Here's how the part is built. I have some questions about the finished solid (model axes, mm). Face numbers are marked on the shaded views. Coordinates: 2 decimals unless noted, no trailing zeros. Write each loop counter-clockwise with the first axis right and the second up, starting at its lowest first coordinate (ties: lowest second). Pieces come first, ordered by that corner, then holes.
Item 1: Please list where these lines run through material, in increasing order: line 1 (X direction, y = 1, z = 51); line 2 (X direction, y = 17.5, z = 131); line 3 (Y direction, x = -18, z = 156).
Item 2: If we mould it in two halves opening along X, with no side actions, what happens to the marked faces 1 and 2? For each: pulls with the +X half, pulls with the -X half, needs draft (parallel to the pull), parting line crosses it, or undercut.
Item 3: I'm going to push flat-ended pins straight in: P1, Ø1.2, axis at y = -18, z = 160, coming from the +X side; P2, Ø12, axis at x = 2.5, y = -11.5, coming from the +Z side; P3, Ø1, axis at x = 11, z = 162.5, coming from the +Y side. Where does each tip first touch, or does it pass through?
Item 4: I want a section at C-C (y = 19). Please give me the cut outline in (x, z), and give its area (3 significant figures).
Item 5: I want a section at B-B (x = 0). Please give me the cut outline in (y, z), and give its area (3 significant figures).
Item 6: I want a section at A-A (y = 1.5). Please give me the cut outline in (x, z), and give its area (3 significant figures).
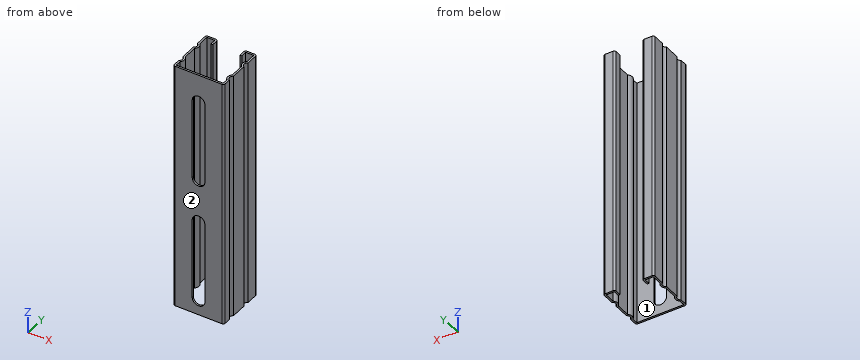
from build123d import *

# Parameters (mm, degrees)
BASE_EXTRUDE_DEPTH = 203.2
SLOT_DEPTH         = 227.830922417
LPATTERN1_COUNT    = 2
LPATTERN1_PITCH    = 101.6


with BuildPart() as part:
    # Sketch1 → Base-Extrude (new body)
    with BuildSketch(Plane.XY):
        with BuildLine():
            Line((-20.6375, 21.1074), (-20.6375, 11.73965134))
            ThreePointArc((-20.6375, 11.73965134), (-19.1389, 9.144), (-20.6375, 6.54834866))
            Line((-20.6375, 6.54834866), (-20.6375, -6.54834866))
            ThreePointArc((-20.6375, -6.54834866), (-19.1389, -9.144), (-20.6375, -11.73965134))
            Line((-20.6375, -11.73965134), (-20.6375, -17.1704))
            ThreePointArc((-20.6375, -17.1704), (-20.198570222, -18.230070222), (-19.1389, -18.669))
            Line((-19.1389, -18.669), (19.1389, -18.669))
            ThreePointArc((19.1389, -18.669), (20.198570222, -18.230070222), (20.6375, -17.1704))
            Line((20.6375, -17.1704), (20.6375, -11.73965134))
            ThreePointArc((20.6375, -11.73965134), (19.1389, -9.144), (20.6375, -6.54834866))
            Line((20.6375, -6.54834866), (20.6375, 6.54834866))
            ThreePointArc((20.6375, 6.54834866), (19.1389, 9.144), (20.6375, 11.73965134))
            Line((20.6375, 11.73965134), (20.6375, 21.1074))
            ThreePointArc((20.6375, 21.1074), (20.198570222, 22.167070222), (19.1389, 22.606))
            Line((19.1389, 22.606), (12.6111, 22.606))
            ThreePointArc((12.6111, 22.606), (11.551429778, 22.167070222), (11.1125, 21.1074))
            Line((11.1125, 21.1074), (11.1125, 16.256))
            Line((11.1125, 16.256), (12.6111, 16.256))
            Line((12.6111, 16.256), (12.6111, 21.1074))
            Line((12.6111, 21.1074), (19.1389, 21.1074))
            Line((19.1389, 21.1074), (19.1389, 12.494971471))
            ThreePointArc((19.1389, 12.494971471), (17.6403, 9.144), (19.1389, 5.793028529))
            Line((19.1389, 5.793028529), (19.1389, -5.793028529))
            ThreePointArc((19.1389, -5.793028529), (17.6403, -9.144), (19.1389, -12.494971471))
            Line((19.1389, -12.494971471), (19.1389, -17.1704))
            Line((19.1389, -17.1704), (-19.1389, -17.1704))
            Line((-19.1389, -17.1704), (-19.1389, -12.494971471))
            ThreePointArc((-19.1389, -12.494971471), (-17.6403, -9.144), (-19.1389, -5.793028529))
            Line((-19.1389, -5.793028529), (-19.1389, 5.793028529))
            ThreePointArc((-19.1389, 5.793028529), (-17.6403, 9.144), (-19.1389, 12.494971471))
            Line((-19.1389, 12.494971471), (-19.1389, 21.1074))
            Line((-19.1389, 21.1074), (-12.6111, 21.1074))
            Line((-12.6111, 21.1074), (-12.6111, 16.256))
            Line((-12.6111, 16.256), (-11.1125, 16.256))
            Line((-11.1125, 16.256), (-11.1125, 21.1074))
            ThreePointArc((-11.1125, 21.1074), (-11.551429778, 22.167070222), (-12.6111, 22.606))
            Line((-12.6111, 22.606), (-19.1389, 22.606))
            ThreePointArc((-19.1389, 22.606), (-20.198570222, 22.167070222), (-20.6375, 21.1074))
        make_face()
    extrude(amount=BASE_EXTRUDE_DEPTH)

    # Sketch2 → Slot (cut, through all)
    with BuildSketch(Plane(origin=(1.121412804, -18.669, -18.780160044), x_dir=(1, 0, 0), z_dir=(0, -1, 0))):
        with BuildLine():
            Line((4.037962196, 97.361410044), (4.037962196, 31.480160044))
            ThreePointArc((4.037962196, 31.480160044), (-1.121412804, 26.320785044), (-6.280787804, 31.480160044))
            Line((-6.280787804, 31.480160044), (-6.280787804, 97.361410044))
            ThreePointArc((-6.280787804, 97.361410044), (-1.121412804, 102.520785044), (4.037962196, 97.361410044))
        make_face()
    slot = extrude(amount=-SLOT_DEPTH, mode=Mode.SUBTRACT)

    # LPattern1: Slot ×2
    with Locations(*[(0, 0, i * LPATTERN1_PITCH) for i in range(1, LPATTERN1_COUNT)]):
        add(slot, mode=Mode.SUBTRACT)


solid = part.part
Answer:
1. line 1: x = -20.64 to -19.14, 19.14 to 20.64
1. line 2: x = -20.64 to -19.14, -12.61 to -11.11, 11.11 to 12.61, 19.14 to 20.64
1. line 3: y = -18.67 to -17.17, -10.91 to -7.38, 7.38 to 10.91, 21.11 to 22.61
2. face 1: undercut
2. face 2: needs draft
3. P1: stops at x = 20.62
3. P2: stops at z = 203.2
3. P3: stops at y = 22.11
4. outline: (-20.64, 0) - (-19.14, 0) - (-19.14, 203.2) - (-20.64, 203.2) - close; (-12.61, 0) - (-11.11, 0) - (-11.11, 203.2) - (-12.61, 203.2) - close; (11.11, 0) - (12.61, 0) - (12.61, 203.2) - (11.11, 203.2) - close; (19.14, 0) - (20.64, 0) - (20.64, 203.2) - (19.14, 203.2) - close
4. area: 1,220 mm2
5. outline: (-18.67, 0) - (-17.17, 0) - (-17.17, 7.54) - (-18.67, 7.54) - close; (-18.67, 83.74) - (-17.17, 83.74) - (-17.17, 109.14) - (-18.67, 109.14) - close; (-18.67, 185.34) - (-17.17, 185.34) - (-17.17, 203.2) - (-18.67, 203.2) - close
5. area: 76.1 mm2
6. outline: (-20.64, 0) - (-19.14, 0) - (-19.14, 203.2) - (-20.64, 203.2) - close; (19.14, 0) - (20.64, 0) - (20.64, 203.2) - (19.14, 203.2) - close
6. area: 609 mm2
